Autodesk Inventor part; units mm, degrees
ref_plane "YZ Plane" through (0, 0, 0) normal (1, 0, 0) x (0, 1, 0)
ref_plane "XZ Plane" through (0, 0, 0) normal (0, 1, 0) x (-1, 0, 0)
ref_plane "XY Plane" through (0, 0, 0) normal (0, 0, 1) x (1, 0, 0)
sketch "Sketch1" plane through (0, 0, 0) normal (0, 1, 0) x (-1, 0, 0)
  line L0 (0, 0) -> (0, -52.7)
  line L1 (0, -52.7) -> (-36, -52.7)
  arc A0 (-36, -52.7) -> (-36, -62.7) centre (-36, -57.7) ccw
  line L2 (-36, -62.7) -> (0, -62.7)
  line L3 (0, -62.7) -> (0, -76)
  line L4 (0, -76) -> (-51, -76)
  line L5 (-51, -76) -> (-51, -23.3)
  line L6 (-51, -23.3) -> (-15, -23.3)
  arc A1 (-15, -23.3) -> (-15, -13.3) centre (-15, -18.3) ccw
  line L7 (-15, -13.3) -> (-51, -13.3)
  line L8 (-51, -13.3) -> (-51, 0)
  line L9 (-51, 0) -> (0, 0)
  point P0 (-25.5, -76)
  dimension "d0" = 76
  dimension "d1" = 10
  dimension "d2" = 10
  dimension "d3" = 29.4
  dimension "d4" = 13.3
  dimension "d17" = 51
  dimension "d18" = 15
  dimension "d19" = 15
extrude "Extrusion1" add sketch "Sketch1" along normal blind 20.5
sketch "Sketch2" plane through (0, 0, 0) normal (0, 0, 1) x (1, 0, 0)
  circle A0 centre (25.5, 10.25) radius 5
  line L0 (0, 0) -> (51, 0)
  line L1 (0, 0) -> (0, 20.5)
  point P0 (25.5, 0)
  point P1 (0, 10.25)
  dimension "d7" = 10
extrude "Extrusion2" cut sketch "Sketch2" against normal up to next
sketch "Sketch3" plane through (51, 0, -76) normal (0, 0, -1) x (-1, 0, 0)
  circle A0 centre (25.5, 10.25) radius 5
  circle A1 centre (25.5, 10.25) radius 5
  point P0 (51, 0)
  point P1 (31.0896, 7.7494)
  point P2 (31.0896, 12.7506)
  point P3 (30.0641, 8.2082)
  point P4 (30.0641, 12.2918)
  dimension "d10" = 5
extrude "Extrusion3" cut sketch "Sketch3" against normal blind 10
sketch "Sketch4" plane through (0, 0, -52.7) normal (-1, 0, 0) x (0, 0, 1)
  line L0 (21.8591, 9.9441) -> (18.2796, 3.7441)
  line L1 (18.2796, 3.7441) -> (11.1204, 3.7441)
  line L2 (11.1204, 3.7441) -> (7.5409, 9.9441)
  line L3 (7.5409, 9.9441) -> (11.1204, 16.1441)
  line L4 (11.1204, 16.1441) -> (18.2796, 16.1441)
  line L5 (18.2796, 16.1441) -> (21.8591, 9.9441)
  line L6 (-23.3, 0) -> (-23.3, 20.5)
  point P0 (52.7, 0)
  point P1 (14.7, 9.9441)
  point P2 (-23.3, 10.25)
  dimension "d13" = 12.4
  dimension "d14" = 38
extrude "Extrusion4" add sketch "Sketch4" along normal blind 10
properties part number "tension_sensor"
Can you work these out from the model? Positions are in its coordinate system, mm. A direction names the side the tool comes from. Coordinates: 2 decimals unless noted, no trailing zeros. Loops run counter-clockwise (first coordinate to the right, second up) from the corner with the lowest first, then second, coordinate; pieces in that order, holes last. Notation, with made-up numbers: (38, 71) - (68, 71) arc R34 cw to (68, 103) - close; hole circle Ø1 at (42.5, 54). An arc over 180 degrees is marked (long way). Use a Markdown table: item, result.
Item 1: Will these pins go through, and if not, where does the flat tip stop? pin 1 (5.5 mm diameter, centred on x = -7, z = -39, fed in from -Y); pin 2 (5 mm diameter, centred on x = 24.5, y = 10, fed in from -Z).
Numbers:
| item | result |
|---|---|
| pin 1 | stops at y = 3.74 |
| pin 2 | stops at z = -66 |
Item 2: I want a section at D-D on x = 37. Please give me the cut outline in (y, z).
Numbers:
| item | result |
|---|---|
| outline | (0, -76) - (20.5, -76) - (20.5, -62.6) - (0, -62.6) - close; (0, -52.8) - (20.5, -52.8) - (20.5, -23.3) - (0, -23.3) - close; (0, -13.3) - (20.5, -13.3) - (20.5, 0) - (0, 0) - close |
Item 3: If I drill on probe 1 along Z at (x, y) = (30.5, 5.75); probe 2 along Y at (x, z) = (25.5, -71.25); probe 3 along Z at (x, y) = (44.5, 8.25), over which ranges is the centre line in solid material (lowest first)? Write a range as from..to.
Numbers:
| item | result |
|---|---|
| probe 1 | z = -76..-62.7, -52.7..-23.3, -13.3..0 |
| probe 2 | y = 0..5.25, 15.25..20.5 |
| probe 3 | z = -76..-23.3, -13.3..0 |
Item 4: I want a section at B-B on y = 7. Please give me the cut outline in (x, z).
Numbers:
| item | result |
|---|---|
| outline | (-10, -43.46) - (0, -43.46) - (0, -52.7) - (36, -52.7) arc R5 cw to (36, -62.7) - (0, -62.7) - (0, -76) - (21.7, -76) - (21.7, -66) - (29.3, -66) - (29.3, -76) - (51, -76) - (51, -23.3) - (15, -23.3) arc R5 cw to (15, -13.3) - (21.7, -13.3) - (21.7, 0) - (0, 0) - (0, -32.54) - (-10, -32.54) - close; (29.3, -13.3) - (51, -13.3) - (51, 0) - (29.3, 0) - close |
Item 5: I want a section at C-C on x = 25.5. Please give me the cut outline in (y, z).
Numbers:
| item | result |
|---|---|
| outline | (0, -76) - (5.25, -76) - (5.25, -66) - (15.25, -66) - (15.25, -76) - (20.5, -76) - (20.5, -62.7) - (0, -62.7) - close; (0, -52.7) - (20.5, -52.7) - (20.5, -23.3) - (0, -23.3) - close; (0, -13.3) - (5.25, -13.3) - (5.25, 0) - (0, 0) - close; (15.25, -13.3) - (20.5, -13.3) - (20.5, 0) - (15.25, 0) - close |
Item 6: We'd pull the mould along X, two halves only. Please class faces 4 (the face through (30.495, 10.47, -71.07)), 5 (the face through (33, 10, -13.3)), 6 (the face through (51, 10, -7)), 7 (the face through (41, 10.1, -57.8)): released by +X, released by -X, zero draft, split by the parting line, or undercut.
Numbers:
| item | result |
|---|---|
| face 4 | undercut |
| face 5 | zero draft |
| face 6 | released by +X |
| face 7 | released by -X |
Item 7: I want a section at A-A on x = 5. Please give me the cut outline in (y, z), and give its area (3 significant figures).
Numbers:
| item | result |
|---|---|
| outline | (0, -76) - (20.5, -76) - (20.5, -62.7) - (0, -62.7) - close; (0, -52.7) - (20.5, -52.7) - (20.5, 0) - (0, 0) - close |
| area | 1,350 mm2 |
Item 8: For faces 1 (the face through (0, 10, -69)), 2 (the face through (26, 10, -66)), 3 (the face through (-4.93, 13.087, -32.656)), which set-ups out of +Z, -Z, +X, -X, +Y, -Y let a thin tool reach every point of the face, with its end or its side?
Numbers:
| item | result |
|---|---|
| face 1 | -Z, -X, +Y, -Y |
| face 2 | -Z |
| face 3 | +Z, -X, +Y |
